Source: CAD feature listing. Evaluate the final solid. Frame: model axes, mm. Coordinates: 2 decimals unless noted, no trailing zeros. Order: outer loops, then holes, each group sorted by start corner. A loop starts at its lowest first (then second) coordinate and runs counter-clockwise, first axis right, second up.
```python
from build123d import *

# Parameters (mm, degrees)
F0_R     = 41
F1_DEPTH = 2
F3_DEPTH = 2.001


with BuildPart() as f1:
    # F0 (on Top) → F1 (new body)
    with BuildSketch(Plane.XY):
        Circle(F0_R)
    extrude(amount=F1_DEPTH)

    # F2 (on face) → F3 (cut, through all)
    with BuildSketch(Plane.XY.offset(2)):
        with BuildLine():
            Line((-23, 0), (-20.5, 0))
            Line((-20.5, 0), (-18.732233047, 1.767766953))
            ThreePointArc((-18.732233047, 1.767766953), (-21.4567085809, 2.3096988313), (-23, 0))
        make_face()
        with BuildLine():
            Line((-18.732233047, -1.767766953), (-20.5, 0))
            Line((-20.5, 0), (-23, 0))
            ThreePointArc((-23, 0), (-21.4567085809, -2.3096988313), (-18.732233047, -1.767766953))
        make_face()
        with BuildLine():
            ThreePointArc((-18.732233047, -1.767766953), (-18.1903011687, -0.9567085809), (-18, 0))
            Line((-18, 0), (-20.5, 0))
            Line((-20.5, 0), (-18.732233047, -1.767766953))
        make_face()
        with BuildLine():
            Line((-20.5, 0), (-18, 0))
            ThreePointArc((-18, 0), (-18.1903011687, 0.9567085809), (-18.732233047, 1.767766953))
            Line((-18.732233047, 1.767766953), (-20.5, 0))
        make_face()
        with BuildLine():
            Line((-1.767766953, 18.732233047), (0, 20.5))
            Line((0, 20.5), (0, 23))
            ThreePointArc((0, 23), (-2.3096988313, 21.4567085809), (-1.767766953, 18.732233047))
        make_face()
        with BuildLine():
            ThreePointArc((-1.767766953, 18.732233047), (-0.9567085809, 18.1903011687), (0, 18))
            Line((0, 18), (0, 20.5))
            Line((0, 20.5), (-1.767766953, 18.732233047))
        make_face()
        with BuildLine():
            Line((0, 20.5), (0, 18))
            ThreePointArc((0, 18), (0.9567085809, 18.1903011687), (1.767766953, 18.732233047))
            Line((1.767766953, 18.732233047), (0, 20.5))
        make_face()
        with BuildLine():
            Line((0, 23), (0, 20.5))
            Line((0, 20.5), (1.767766953, 18.732233047))
            ThreePointArc((1.767766953, 18.732233047), (2.3096988313, 19.5432914191), (2.5, 20.5))
            ThreePointArc((2.5, 20.5), (1.767766953, 22.267766953), (0, 23))
        make_face()
        with BuildLine():
            Line((-4.772970773, 4.772970773), (0, 0))
            Line((0, 0), (0, 6.75))
            ThreePointArc((0, 6.75), (-2.5831131685, 6.2361868445), (-4.772970773, 4.772970773))
        make_face()
        with BuildLine():
            Line((-6.75, 0), (0, 0))
            Line((0, 0), (-4.772970773, 4.772970773))
            ThreePointArc((-4.772970773, 4.772970773), (-6.2361868445, 2.5831131685), (-6.75, 0))
        make_face()
        with BuildLine():
            Line((-4.772970773, -4.772970773), (0, 0))
            Line((0, 0), (-6.75, 0))
            ThreePointArc((-6.75, 0), (-6.2361868445, -2.5831131685), (-4.772970773, -4.772970773))
        make_face()
        with BuildLine():
            Line((0, -6.75), (0, 0))
            Line((0, 0), (-4.772970773, -4.772970773))
            ThreePointArc((-4.772970773, -4.772970773), (-2.5831131685, -6.2361868445), (0, -6.75))
        make_face()
        with BuildLine():
            Line((4.772970773, -4.772970773), (0, 0))
            Line((0, 0), (0, -6.75))
            ThreePointArc((0, -6.75), (2.5831131685, -6.2361868445), (4.772970773, -4.772970773))
        make_face()
        with BuildLine():
            Line((6.75, 0), (0, 0))
            Line((0, 0), (5.7423592933, -3.5479303469))
            ThreePointArc((5.7423592933, -3.5479303469), (6.4932051111, -1.8441223888), (6.75, 0))
        make_face()
        with BuildLine():
            Line((5.7423592933, 3.5479303469), (0, 0))
            Line((0, 0), (6.75, 0))
            ThreePointArc((6.75, 0), (6.4932051111, 1.8441223888), (5.7423592933, 3.5479303469))
        make_face()
        with BuildLine():
            Line((0, 6.75), (0, 0))
            Line((0, 0), (4.772970773, 4.772970773))
            ThreePointArc((4.772970773, 4.772970773), (2.5831131685, 6.2361868445), (0, 6.75))
        make_face()
        with BuildLine():
            Line((5.7423592933, -3.5479303469), (0, 0))
            Line((0, 0), (4.772970773, -4.772970773))
            ThreePointArc((4.772970773, -4.772970773), (5.2932242171, -4.1885889495), (5.7423592933, -3.5479303469))
        make_face()
        with BuildLine():
            Line((4.772970773, 4.772970773), (0, 0))
            Line((0, 0), (5.7423592933, 3.5479303469))
            ThreePointArc((5.7423592933, 3.5479303469), (5.2932242171, 4.1885889495), (4.772970773, 4.772970773))
        make_face()
        with BuildLine():
            Line((0, -23), (0, -20.5))
            Line((0, -20.5), (-1.767766953, -18.732233047))
            ThreePointArc((-1.767766953, -18.732233047), (-2.3096988313, -21.4567085809), (0, -23))
        make_face()
        with BuildLine():
            ThreePointArc((1.767766953, -18.732233047), (0.9567085809, -18.1903011687), (0, -18))
            Line((0, -18), (0, -20.5))
            Line((0, -20.5), (1.767766953, -18.732233047))
        make_face()
        with BuildLine():
            Line((0, -20.5), (0, -18))
            ThreePointArc((0, -18), (-0.9567085809, -18.1903011687), (-1.767766953, -18.732233047))
            Line((-1.767766953, -18.732233047), (0, -20.5))
        make_face()
        with BuildLine():
            Line((1.767766953, -18.732233047), (0, -20.5))
            Line((0, -20.5), (0, -23))
            ThreePointArc((0, -23), (1.767766953, -22.267766953), (2.5, -20.5))
            ThreePointArc((2.5, -20.5), (2.3096988313, -19.5432914191), (1.767766953, -18.732233047))
        make_face()
        with BuildLine():
            Line((41, 0), (31, 0))
            Line((31, 0), (31, -26.83281573))
            ThreePointArc((31, -26.83281573), (38.4187454246, -14.3178210633), (41, 0))
        make_face()
        with BuildLine():
            Line((31, 26.83281573), (31, 0))
            Line((31, 0), (41, 0))
            ThreePointArc((41, 0), (38.4187454246, 14.3178210633), (31, 26.83281573))
        make_face()
    extrude(amount=-F3_DEPTH, mode=Mode.SUBTRACT)


solid = f1.part
```
1. Section query C-C on x = 15. Return loops of the section in (y, z), plus the area to 3 significant figures.
Findings:
outline: (-38.16, 0) - (38.16, 0) - (38.16, 2) - (-38.16, 2) - close
area: 153 mm2
2. Section query A-A on z = 1.45. Return loops of the section in (x, y), plus the area to 3 significant figures.
Findings:
outline: (31, -26.83) - (31, 26.83) arc R41 ccw (long way) to start; hole circle Ø5 at (-20.5, 0); hole circle Ø13.5 at (0, 0); hole circle Ø5 at (0, -20.5); hole circle Ø5 at (0, 20.5)
area: 4,710 mm2
3. Pin query (flat end, axial travel): P1, Ø4, axis at x = 2, y = 5, coming from the +Z side. Return the tip coordinate at first contact, or that it passes through.
Findings:
P1: stops at z = 2
4. Section query D-D on y = 31. Return loops of the section in (x, z).
Findings:
outline: (-26.83, 0) - (26.83, 0) - (26.83, 2) - (-26.83, 2) - close
5. Section query B-B on y = -21.5. Return loops of the section in (x, z).
Findings:
outline: (-34.91, 0) - (-2.29, 0) - (-2.29, 2) - (-34.91, 2) - close; (2.29, 0) - (31, 0) - (31, 2) - (2.29, 2) - close
6. Ray query, line 1 (X direction, y = -1.5, z = 1.35); line 2 (Y direction, x = 5, z = 1.7); line 3 (Y direction, x = 1, z = 1.4). Return the intervals inside material, ascending.
Findings:
line 1: x = -40.97 to -22.5, -18.5 to -6.58, 6.58 to 31
line 2: y = -40.69 to -4.53, 4.53 to 40.69
line 3: y = -40.99 to -22.79, -18.21 to -6.68, 6.68 to 18.21, 22.79 to 40.99
